Geometry check sheet. Reference: drawing and pictorial views, mm from the part's lowest x, y, z. A direction names the side the tool comes from. Round coordinates to 2 decimals unless told otherwise and drop trailing zeros. Write each loop counter-clockwise with the first axis right and the second up, starting at its lowest first coordinate (ties: lowest second). Pieces come first, ordered by that corner, then holes. Notation, with made-up numbers: (-14.75, 18) - (34.25, 18) arc R18 ccw to (34.25, 37) - close; hole circle Ø7 at (37, 66.5). An arc over 180 degrees is marked (long way). Return JSON: item names as keys, results as strings.
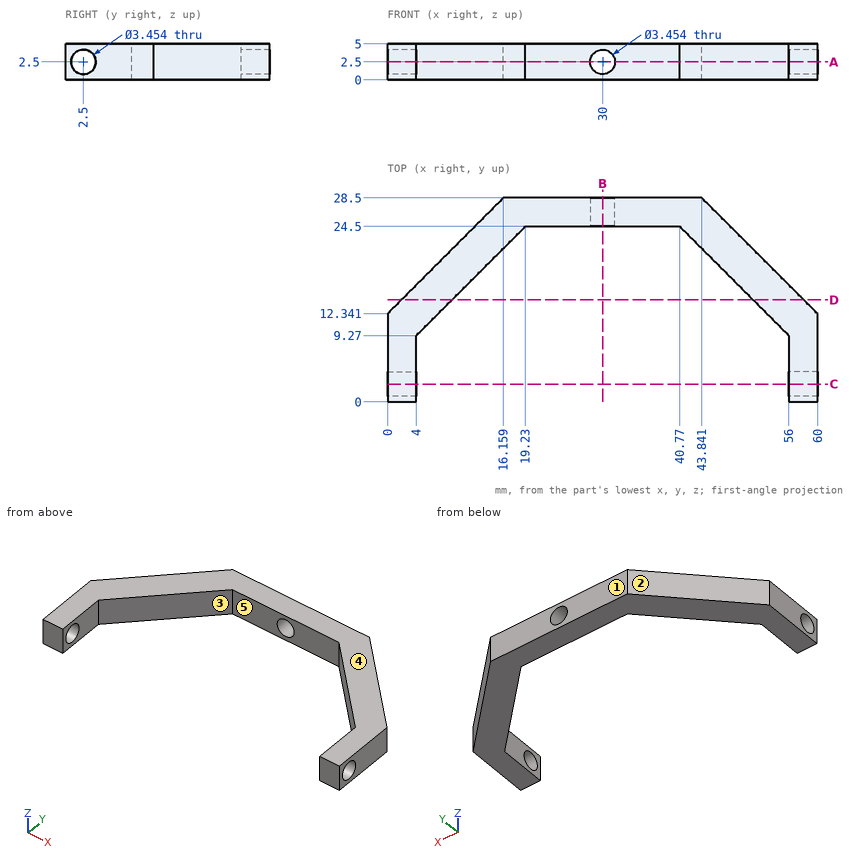
(1) Material ranges on line 1 along Z through (x, y) = (30, 26.6); line 2 along X through (y, z) = (5.25, 2.35); line 3 along X through (y, z) = (19.25, 2.8), recorded low to high. Write a range as [from, to].
Response values:
{"line 1": "z = [0, 0.77], [4.23, 5]", "line 2": "x = [0, 4], [56, 60]", "line 3": "x = [6.91, 13.98], [46.02, 53.09]"}
(2) Access from +Z, -Z, +X, -X, +Y, -Y to the whole of each face (thin tool, end or side, straight path). Record for the marked faces 4 and 5.
Response values:
{"face 4": "+Z, +X, -X, +Y, -Y", "face 5": "+Z, -Z, -Y"}
(3) Section check D-D, the plane y = 14.25. Enter the section's corners in (x, z).
Response values:
{"outline": "(1.91, 0) - (8.98, 0) - (8.98, 5) - (1.91, 5) - close; (51.02, 0) - (58.09, 0) - (58.09, 5) - (51.02, 5) - close"}
(4) Gauge pin test, flat end, axial feed: pin 1 (2.5 mm diameter, centred on x = 29, z = 1.5, fed in from -Y). Record the tip position at first contact, or that the pin passes through.
Response values:
{"pin 1": "stops at y = 24.5"}
(5) Release check for a two-part mould opening along X. For the marked faces 1, 2 and 3 record: pulls with the +X half, pulls with the -X half, needs draft (parallel to the pull), parting line crosses it, or undercut.
Response values:
{"face 1": "needs draft", "face 2": "pulls with the -X half", "face 3": "undercut"}
(6) Section check B-B, the plane x = 30. Enter the section's corners in (y, z).
Response values:
{"outline": "(24.5, 0) - (28.5, 0) - (28.5, 0.77) - (24.5, 0.77) - close; (24.5, 4.23) - (28.5, 4.23) - (28.5, 5) - (24.5, 5) - close"}
(7) Section check C-C, the plane y = 2.5. Enter the section's corners in (x, z).
Response values:
{"outline": "(0, 0) - (4, 0) - (4, 0.77) - (0, 0.77) - close; (0, 4.23) - (4, 4.23) - (4, 5) - (0, 5) - close; (56, 0) - (60, 0) - (60, 0.77) - (56, 0.77) - close; (56, 4.23) - (60, 4.23) - (60, 5) - (56, 5) - close"}
(8) Section check A-A, the plane z = 2.5. Enter the section's corners in (x, y).
Response values:
{"outline": "(0, 0) - (4, 0) - (4, 0.77) - (0, 0.77) - close; (0, 4.23) - (4, 4.23) - (4, 9.27) - (19.23, 24.5) - (28.27, 24.5) - (28.27, 28.5) - (16.16, 28.5) - (0, 12.34) - close; (31.73, 24.5) - (40.77, 24.5) - (56, 9.27) - (56, 4.23) - (60, 4.23) - (60, 12.34) - (43.84, 28.5) - (31.73, 28.5) - close; (56, 0) - (60, 0) - (60, 0.77) - (56, 0.77) - close"}
